from build123d import *

# Parameters (mm, degrees)
BOSS_EXTRUDE1_DEPTH = 10
CUT_EXTRUDE1_REACH  = 46.811
SKETCH2_R           = 2
CUT_EXTRUDE2_START  = -3
CUT_EXTRUDE2_DEPTH  = 36


with BuildPart() as part:
    # Sketch1 → Boss-Extrude1 (new body)
    with BuildSketch(Plane(origin=(0, 0, 0), x_dir=(1, 0, 0), z_dir=(0, 1, 0))):
        with BuildLine():
            Line((16, -12), (-16, -12))
            ThreePointArc((-16, -12), (-19.535533906, -10.535533906), (-21, -7))
            Line((-21, -7), (-21, 7))
            ThreePointArc((-21, 7), (-19.535533906, 10.535533906), (-16, 12))
            Line((-16, 12), (16, 12))
            ThreePointArc((16, 12), (19.535533906, 10.535533906), (21, 7))
            Line((21, 7), (21, -7))
            ThreePointArc((21, -7), (19.535533906, -10.535533906), (16, -12))
        make_face()
        with BuildLine():
            Line((-10, -6), (10, -6))
            ThreePointArc((10, -6), (13.535533906, -4.535533906), (15, -1))
            Line((15, -1), (15, 1))
            ThreePointArc((15, 1), (13.535533906, 4.535533906), (10, 6))
            Line((10, 6), (-10, 6))
            ThreePointArc((-10, 6), (-13.535533906, 4.535533906), (-15, 1))
            Line((-15, 1), (-15, -1))
            ThreePointArc((-15, -1), (-13.535533906, -4.535533906), (-10, -6))
        make_face(mode=Mode.SUBTRACT)
    extrude(amount=BOSS_EXTRUDE1_DEPTH)

    # Cut-Extrude1: up to this face of the body (flat: up to its plane)
    cut_extrude1_end = Plane(part.part.faces().sort_by_distance((-21, 5, 0))[0])
    # Sketch2 → Cut-Extrude1 (cut, up to the picked face)
    with BuildSketch(Plane(origin=(21, 0, 0), x_dir=(0, 0, -1), z_dir=(1, 0, 0)), mode=Mode.PRIVATE) as cut_extrude1_sk1:
        with Locations((0, 5)):
            Circle(SKETCH2_R)
    cut_extrude1_tool1 = split(extrude(cut_extrude1_sk1.sketch, amount=-CUT_EXTRUDE1_REACH, mode=Mode.PRIVATE), bisect_by=cut_extrude1_end, keep=Keep.BOTH, mode=Mode.PRIVATE)
    add(cut_extrude1_tool1.solids().sort_by(Axis((21, 5, 0), (-1, 0, 0)))[0], mode=Mode.SUBTRACT)

    # Sketch3 → Cut-Extrude2 (cut)
    with BuildSketch(Plane(origin=(-15, 0, 0), x_dir=(0, 0, -1), z_dir=(1, 0, 0)).offset(CUT_EXTRUDE2_START)):
        Polygon((3.464101615, 5), (1.732050808, 8), (-1.732050808, 8), (-3.464101615, 5), (-1.732050808, 2), (1.732050808, 2), align=None)
    extrude(amount=CUT_EXTRUDE2_DEPTH, mode=Mode.SUBTRACT)


solid = part.part
CAD build for the part. Positions are in the model's coordinates, mm. A direction names the side the tool comes from. Give positions to 0.01 mm unless a question says otherwise; leave off trailing zeros. Loops run counter-clockwise (first coordinate to the right, second up) from the corner with the lowest first, then second, coordinate; pieces in that order, holes last. Notation, with made-up numbers: M 20.25,-8.5 L 53.25,-8.5 A25 cw 53.25,28.5 Z; hole C 33.5,27.25 d7. An arc over 180 degrees is marked long. Answer in a Markdown table with one row per item. Add a question column.
Item 1: Mould opens along Y. For faces 1 (the face through (19, 5, -11)), 2 (the face through (-16, 8, 0)), 3 (the face through (0, 0, -8)) say: +Y half, -Y half, draft (parallel to the pull), parting line (faces both ways), or undercut.
Item 2: Band-saw the part on B-B on x = 9.5. Give the cut face in (y, z).
Item 3: Band-saw the part on A-A on z = 0. Give the cut face in (x, y), then the cut area to 3 significant figures.
Item 4: Tool access for faces 4 (the face through (-18, 7, -1)), 5 (the face through (0, 5, -6)), 6 (the face through (20, 5, 10)): list every direction of +Z, -Z, +X, -X, +Y, -Y with a clear straight run to the whole face (end or side of a thin tool).
Item 5: Band-saw the part on D-D on y = 9. Give the cut face in (x, z).
Item 6: Drop flat-ended pins along their axis: P1, Ø2.5, axis at y = 5, z = 0, coming from the +X side; P2, Ø1.8, axis at y = 3.5, z = 0.5, coming from the +X side. Give the stop position or say it passes through.
Item 7: Probe probe 1 along Y at (x, z) = (-18.65, 0); probe 2 along Z at (x, y) = (1.5, 7.5); probe 3 along Y at (x, z) = (-17, 0.5). List the from-to ranges inside material, lowest first.
Item 8: Band-saw the part on C-C on z = 5. Give the cut face in (x, y).
Reply:
| question | item | result |
|---|---|---|
| 1 | face 1 | draft |
| 1 | face 2 | undercut |
| 1 | face 3 | -Y half |
| 2 | outline | M 0,-12 L 10,-12 L 10,-6 L 0,-6 Z; M 0,6 L 10,6 L 10,12 L 0,12 Z |
| 3 | outline | M -21,0 L -15,0 L -15,2 L -18,2 L -18,3 L -21,3 Z; M -21,7 L -18,7 L -18,8 L -15,8 L -15,10 L -21,10 Z; M 15,0 L 21,0 L 21,3 L 18,3 L 18,2 L 15,2 Z; M 15,8 L 18,8 L 18,7 L 21,7 L 21,10 L 15,10 Z |
| 3 | area | 60.0 mm^2 |
| 4 | face 4 | none |
| 4 | face 5 | +Y, -Y |
| 4 | face 6 | +Z, +X, +Y, -Y |
| 5 | outline | M -21,-7 A5 ccw -16,-12 L 16,-12 A5 ccw 21,-7 L 21,7 A5 ccw 16,12 L -16,12 A5 ccw -21,7 Z; hole M -15,-1 A5 ccw -10,-6 L 10,-6 A5 ccw 15,-1 L 15,1 A5 ccw 10,6 L -10,6 A5 ccw -15,1 Z |
| 6 | P1 | passes through |
| 6 | P2 | stops at x = 21 |
| 7 | probe 1 | y = 0 to 3, 7 to 10 |
| 7 | probe 2 | z = -12 to -6, 6 to 12 |
| 7 | probe 3 | y = 0 to 2, 8 to 10 |
| 8 | outline | M -21,0 L -13,0 L -13,10 L -21,10 Z; M 13,0 L 21,0 L 21,10 L 13,10 Z |
